from build123d import *

# Parameters (mm, degrees)
F1_R     = 31.75
F1_R_2   = 19.05
F4_DEPTH = 50.8
F2_R     = 19.05
F2_R_2   = 12.7
F5_DEPTH = 38.1
F6_DEPTH = 19.05
F3_R     = 9.525
F7_DEPTH = 19.05


with BuildPart() as f4:
    # F1 (on Top) → F4 (new body)
    with BuildSketch(Plane.XY):
        Circle(F1_R)
        Circle(F1_R_2, mode=Mode.SUBTRACT)
    extrude(amount=F4_DEPTH)

    # F2 (on face) → F5 (join)
    with BuildSketch(Plane.XY):
        Circle(F2_R)
        Circle(F2_R_2, mode=Mode.SUBTRACT)
    extrude(amount=F5_DEPTH)

    # F0 (on Top) → F6 (join)
    with BuildSketch(Plane.XY):
        with BuildLine():
            ThreePointArc((18.9071120655, 25.5065405992), (28.3580967986, 14.2786850221), (31.75, 0))
            ThreePointArc((31.75, 0), (28.3738258286, -14.2474035476), (18.9633223402, -25.4647777493))
            Line((18.9633223402, -25.4647777493), (74.598514582, -25.4647777493))
            ThreePointArc((74.598514582, -25.4647777493), (98.1416650574, 1.2092358238), (72.1527459753, 25.5065405992))
            Line((72.1527459753, 25.5065405992), (18.9071120655, 25.5065405992))
        make_face()
        with BuildLine():
            ThreePointArc((45.1813528665, -9.5272837666), (35.1847662251, -0.3951371067), (44.4197335774, 9.5065407864))
            Line((44.4197335774, 9.5065407864), (72.3597335774, 9.5065407864))
            ThreePointArc((72.3597335774, 9.5065407864), (82.1679704992, 0.1258636982), (72.6398616433, -9.5392154931))
            Line((72.6398616433, -9.5392154931), (45.1813528665, -9.5272837666))
        make_face(mode=Mode.SUBTRACT)
    extrude(amount=F6_DEPTH)

    # F3 (on face) → F7 (join)
    with BuildSketch(Plane.XY):
        with BuildLine():
            Line((-49.5730978943, -25.4974987052), (-18.9193038925, -25.4974987052))
            ThreePointArc((-18.9193038925, -25.4974987052), (-31.7478647233, -0.3682193799), (-19.5055872667, 25.0518375649))
            Line((-19.5055872667, 25.0518375649), (-50.4100229924, 25.5240209789))
            ThreePointArc((-50.4100229924, 25.5240209789), (-76.3235664091, -0.41867262), (-49.5730978943, -25.4974987052))
        make_face()
        with Locations((-50.8, 0)):
            Circle(F3_R, mode=Mode.SUBTRACT)
    extrude(amount=F7_DEPTH)


solid = f4.part
Read the model definition and answer for the solid it produces. Units are mm, in the model's axes. A direction names the side the tool comes from. Round coordinates to 2 decimals unless told otherwise and drop trailing zeros. Order: outer loops, then holes, each group sorted by start corner. A loop starts at its lowest first (then second) coordinate and runs counter-clockwise, first axis right, second up. Notation, with made-up numbers: (-35.75, 5) - (-18.75, 5) arc R24 cw to (-18.75, 43) - close; hole circle Ø10 at (47, 32). An arc over 180 degrees is marked (long way). Use one line per item in the form item = value. Start each with the question number.
(1) The part is cut by section B-B (y = -7). Give the vertices of the cut face in (x, z).
(2) The part is cut by section A-A (z = 15). Count the separate pieces of the cut face and the enclosed holes in it, then the cut area to 3 significant figures.
(3) For faces 1 (the face through (14, -14, 50.8)), 2 (the face through (46, 25.507, 9)), 3 (the face through (46, -25.465, 9)), 4 (the face through (82.163, 0.337, 9.392)), 5 (the face through (4, -12.4, 38.1)), determine the directions among +Z, -Z, +X, -X, +Y, -Y from which every point of the face is accessible in a straight line to the end or side of a thin tool.
(4) The part is cut by section C-C (x = 0). Give the vertices of the cut face in (y, z), then the cut area to 3 significant figures.
(5) Flat-ended cylindrical pins translate along their axes: pin 1 Ø5 at (y, z) = (13, 34.5) entering from +X; pin 2 Ø5 at (y, z) = (6.5, 41.5) entering from +X; pin 3 Ø4 at (y, z) = (-2, 30.5) entering from +X. Find the tip coordinate at first contact, or state that the pin passes through.
(6) The part is cut by section D-D (z = 26.5). Give the vertices of the cut face in (x, y), then the cut area to 3 significant figures.
(7) Find the intervals of material crossed by line 1 along Y through (x, z) = (0, 9); line 2 along Y through (x, z) = (-50.8, 6.75) (3 decimals); line 3 along Z through (x, y) = (90.5, 9.5), in increasing order. Write a range as from..to.
Checked values:
q1.outline = (-75.35, 0) - (-57.26, 0) - (-57.26, 19.05) - (-75.35, 19.05) - close; (-44.34, 0) - (-10.6, 0) - (-10.6, 38.1) - (-17.72, 38.1) - (-17.72, 50.8) - (-30.97, 50.8) - (-30.97, 19.05) - (-44.34, 19.05) - close; (10.6, 0) - (38.23, 0) - (38.23, 19.05) - (30.97, 19.05) - (30.97, 50.8) - (17.72, 50.8) - (17.72, 38.1) - (10.6, 38.1) - close; (79.12, 0) - (97.2, 0) - (97.2, 19.05) - (79.12, 19.05) - close
q2.separate_pieces = 1
q2.enclosed_holes = 3
q2.area = 7,050 mm^2
q3.face_1 = +Z, +X, -X, +Y, -Y
q3.face_2 = +Z, -Z, +X, +Y
q3.face_3 = +Z, -Z, +X, -Y
q3.face_4 = +Z, -Z
q3.face_5 = +Z
q4.outline = (-31.75, 0) - (-12.7, 0) - (-12.7, 38.1) - (-19.05, 38.1) - (-19.05, 50.8) - (-31.75, 50.8) - close; (12.7, 0) - (31.75, 0) - (31.75, 50.8) - (19.05, 50.8) - (19.05, 38.1) - (12.7, 38.1) - close
q4.area = 1,770 mm^2
q5.pin_1 = 29.96
q5.pin_2 = 31.5
q5.pin_3 = 31.75
q6.outline = circle Ø63.5 at (0, 0); hole circle Ø25.4 at (0, 0)
q6.area = 2,660 mm^2
q7.line_1 = -31.75..-12.7, 12.7..31.75
q7.line_2 = -25.527..-9.525, 9.525..25.527
q7.line_3 = 0..19.05
